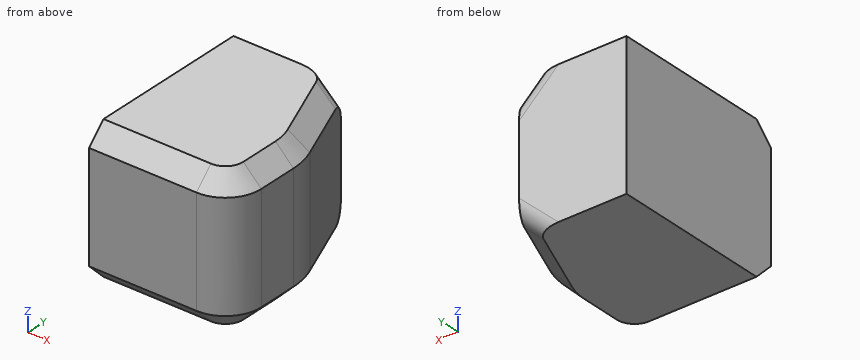
```python
from build123d import *

# Parameters (mm, degrees)
BOSS_EXTRUDE2_DEPTH = 40
CHAMFER2_SIZE       = 5
FILLET2_R           = 5


with BuildPart() as part:
    # Sketch2 → Boss-Extrude2 (new body)
    with BuildSketch(Plane.XY):
        with BuildLine():
            Line((0, 0), (0, 50))
            Line((0, 50), (30, 50))
            Line((30, 50), (38.569533818, 28.576165456))
            ThreePointArc((38.569533818, 28.576165456), (39.639127735, 24.930502352), (40, 21.148351929))
            Line((40, 21.148351929), (40, 10))
            ThreePointArc((40, 10), (37.071067812, 2.928932188), (30, 0))
            Line((30, 0), (0, 0))
        make_face()
    extrude(amount=BOSS_EXTRUDE2_DEPTH)

    # Chamfer2
    chamfer2_edges = [part.edges().sort_by_distance(p)[0] for p in [
        (15, 0, 0),
        (40, 15.574175964, 40),
        (39.639127735, 24.930502352, 40),
        (34.284766909, 39.288082728, 40),
        (15, 0, 40),
        (34.284766909, 39.288082728, 0),
        (39.639127735, 24.930502352, 0),
        (37.071067812, 2.928932188, 40),
        (40, 15.574175964, 0),
        (37.071067812, 2.928932188, 0),
    ]]
    chamfer(chamfer2_edges, length=CHAMFER2_SIZE)

    # Fillet2
    fillet2_edges = [part.edges().sort_by_distance(p)[0] for p in [
        (27.307417596, 50, 37.5),
        (27.307417596, 50, 2.5),
    ]]
    fillet(fillet2_edges, radius=FILLET2_R)


solid = part.part
```
Geometry check sheet. Reference: the model listing, model coordinates, mm. Coordinates: 2 decimals unless noted, no trailing zeros. Order: outer loops, then holes, each group sorted by start corner. A loop starts at its lowest first (then second) coordinate and runs counter-clockwise, first axis right, second up. Notation, with made-up numbers: M -34.75,47.25 L 13.25,47.25 A21 cw 13.25,75.25 Z; hole C 89,-14.75 d3. An arc over 180 degrees is marked long. Answer as a JSON object with one key per item and string values.
Q1. Cross-section at B-B on y = 13. Record the cut outline in (x, z), and give its area (4 significant figures).
Results are:
{"outline": "M 0,0 L 35,0 L 40,5 L 40,35 L 35,40 L 0,40 Z", "area": "1,575 mm²"}
Q2. Cross-section at A-A on z = 13.5. Record the cut outline in (x, y), and give its area (3 significant figures).
Results are:
{"outline": "M 0,0 L 30,0 A10 ccw 40,10 L 40,21.15 A20 ccw 38.57,28.58 L 30,50 L 0,50 Z", "area": "1,850 mm²"}
Q3. Scan lines: line 1 (Y direction, x = 6, z = 37.5); line 2 (Y direction, x = 15, z = 36.5); line 3 (X direction, y = 29, z = 21). Record each from-to range of solid material in increasing order.
Results are:
{"line 1": "y = 2.5 to 50", "line 2": "y = 1.5 to 50", "line 3": "x = 0 to 38.4"}
Q4. Cross-section at C-C on y = 38. Record the cut outline in (x, z), and give its area (3 significant figures).
Results are:
{"outline": "M 0,0 L 29.41,0 L 34.8,5 L 34.8,35 L 29.41,40 L 0,40 Z", "area": "1,370 mm²"}
